Input: part model. Units: mm. Frame: model coordinates. A direction names the side the tool comes from. Coordinates: 2 decimals unless noted, no trailing zeros. Order: outer loops, then holes, each group sorted by start corner. A loop starts at its lowest first (then second) coordinate and runs counter-clockwise, first axis right, second up. Notation, with made-up numbers: (-27.5, 45.25) - (-20.5, 45.25) arc R14 cw to (-20.5, 62.25) - close; hole circle Ø3 at (-14, 6.5). An arc over 180 degrees is marked (long way). Use a Markdown table: item, result. Add a question column.
Autodesk Inventor part; units mm, degrees
ref_plane "YZ Plane" through (0, 0, 0) normal (1, 0, 0) x (0, 1, 0)
ref_plane "XZ Plane" through (0, 0, 0) normal (0, 1, 0) x (-1, 0, 0)
ref_plane "XY Plane" through (0, 0, 0) normal (0, 0, 1) x (1, 0, 0)
sketch "Sketch1" plane through (0, 0, 0) normal (0, 0, 1) x (1, 0, 0)
  line L0 (0, 0) -> (22.352, 0)
  line L1 (22.352, 0) -> (22.352, 36.83)
  line L2 (22.352, 36.83) -> (0, 36.83)
  line L3 (0, 36.83) -> (0, 0)
  dimension "d0" = 22.352
  dimension "d1" = 36.83
extrude "Extrusion1" add sketch "Sketch1" along normal blind 20.828
sketch "Sketch2" plane through (0, 36.83, 0) normal (0, 1, 0) x (1, 0, 0)
  circle A0 centre (11.176, -10.414) radius 8.509
  point P0 (0, 0)
  dimension "d4" = 17.018
extrude "Extrusion2" add sketch "Sketch2" along normal blind 25.4
sketch "Sketch3" plane through (0, 0, 0) normal (0, 0, -1) x (-1, 0, 0)
  point P0 (0, 0)
sketch "Sketch4" plane through (0, 0, 20.828) normal (0, 0, 1) x (1, 0, 0)
  line L0 (22.352, 36.83) -> (0, 36.83)
  line L1 (0, 36.83) -> (0, 0)
  circle A0 centre (2.2352, 30.734) radius 1.27
  line L2 (22.352, 0) -> (22.352, 36.83)
  circle A1 centre (20.1168, 30.734) radius 1.27
  dimension "d9" = 2.54
  dimension "d12" = 2.54
extrude "Extrusion3" cut sketch "Sketch4" against normal blind 25.4
sketch "Sketch5" plane through (0, 0, 0) normal (0, 0, -1) x (-1, 0, 0)
  point P0 (0, 0)
sketch "Sketch6" plane through (0, 0, 20.828) normal (0, 0, 1) x (1, 0, 0)
  line L0 (0, 0) -> (22.352, 0)
  line L1 (11.176, 0) -> (11.176, 7.62)
  line L2 (22.352, 0) -> (22.352, 11.43)
  line L3 (22.352, 11.43) -> (13.589, 11.43)
  line L4 (0, 11.43) -> (8.763, 11.43)
  line L5 (13.589, 8.5992) -> (13.589, 14.2608)
  line L6 (8.763, 14.3275) -> (8.763, 8.5325)
  line L7 (8.763, 7.6515) -> (13.589, 15.2085) construction
  line L8 (13.589, 7.6515) -> (8.763, 15.2085) construction
  arc A0 (8.763, 8.5325) -> (13.589, 8.5992) centre (11.14, 11.1716) ccw
  arc A1 (13.589, 14.2608) -> (8.763, 14.3275) centre (11.14, 11.6884) ccw
  point P0 (11.176, 11.43)
  dimension "d16" = 7.62
  dimension "d17" = 11.43
  dimension "d18" = 8.763
extrude "Extrusion4" add sketch "Sketch6" along normal blind 5.334 contours A0 L6 A1 L5
properties part number "msheehan_motor"
1) Pull-direction query (X, two-part tool) for faces 1 (the cylindrical face through (11.23, 7.62, 23.46)), 2 (the cylindrical face through (18.85, 30.79, 10.56)), 3 (the flat face through (11, 19, 20.828)); classes: pulls with the +X half, pulls with the -X half, needs draft (parallel to the pull), parting line crosses it, or undercut.
2) Cut plane C-C (y = 27.5). Return the cut outline in (x, z).
3) Material intervals for L1, parallel to Y at x = 20.25, z = 6.75; L2, parallel to Z at x = 15.75, y = 20.5; L3, parallel to X at y = 53, z = 10.5, sorted ascending.
4) Contact query for flat-ended pins moving along their axis: P1, Ø5, axis at y = 44.5, z = 9.5, coming from the -X side; P2, Ø6, axis at x = 16, y = 48, coming from the +Z side; P3, Ø8, axis at x = 9, y = 29, coming from the +Z side. Output: stop coordinate, or through.
5) Cut plane A-A (z = 11.5). Return the cut outline in (x, y), and give its area (3 significant figures).
6) Reachability of faces 4 (the flat face through (0, 19, 10)), 5 (the cylindrical face through (11.15, 15.24, 23.46)), 6 (the cylindrical face through (2.675, 49.352, 10.788)), 7 (the flat face through (8.763, 11, 23)), 8 (the flat face through (13.589, 11, 23)) from +Z, -Z, +X, -X, +Y, -Y: full face, straight path, thin tool, end or side. Return the list, or none.
7) Cut plane B-B (x = 14.5). Return the cut outline in (y, z), and give its area (3 significant figures).
8) Cut plane D-D (z = 2.75). Return the cut outline in (x, y), and give its area (3 significant figures).
Computed:
| question | item | result |
|---|---|---|
| 1 | face 1 | parting line crosses it |
| 1 | face 2 | undercut |
| 1 | face 3 | needs draft |
| 2 | outline | (0, 0) - (22.35, 0) - (22.35, 20.83) - (0, 20.83) - close |
| 3 | L1 | y = 0 to 29.47, 32 to 36.83 |
| 3 | L2 | z = 0 to 20.83 |
| 3 | L3 | x = 2.67 to 19.68 |
| 4 | P1 | stops at x = 2.67 |
| 4 | P2 | stops at z = 18.73 |
| 4 | P3 | stops at z = 20.83 |
| 5 | outline | (0, 0) - (22.35, 0) - (22.35, 36.83) - (19.62, 36.83) - (19.62, 62.23) - (2.74, 62.23) - (2.74, 36.83) - (0, 36.83) - close; hole circle Ø2.54 at (2.24, 30.73); hole circle Ø2.54 at (20.12, 30.73) |
| 5 | area | 1,240 mm2 |
| 6 | face 4 | +Z, -Z, -X, +Y, -Y |
| 6 | face 5 | +Z, +Y |
| 6 | face 6 | +Y |
| 6 | face 7 | +Z, -X, +Y, -Y |
| 6 | face 8 | +Z, +X, +Y, -Y |
| 7 | outline | (0, 0) - (36.83, 0) - (36.83, 2.58) - (62.23, 2.58) - (62.23, 18.25) - (36.83, 18.25) - (36.83, 20.83) - (0, 20.83) - close |
| 7 | area | 1,170 mm2 |
| 8 | outline | (0, 0) - (22.35, 0) - (22.35, 36.83) - (14.87, 36.83) - (14.87, 62.23) - (7.48, 62.23) - (7.48, 36.83) - (0, 36.83) - close; hole circle Ø2.54 at (2.24, 30.73); hole circle Ø2.54 at (20.12, 30.73) |
| 8 | area | 1,000 mm2 |
